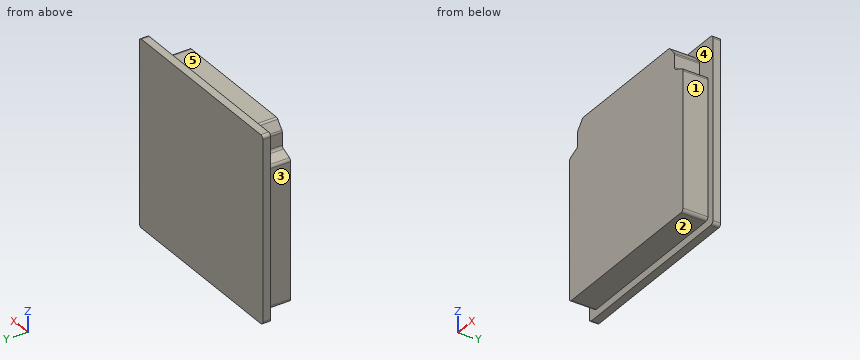
```python
from build123d import *

# Parameters (mm, degrees)
F0_W     = 29.8
F0_H     = 29.8
F1_DEPTH = 1.25
F3_DEPTH = 4
F4_R     = 0.5


with BuildPart() as f1:
    # F0 (on Front) → F1 (new body)
    with BuildSketch(Plane.XZ):
        Rectangle(F0_W, F0_H)
    extrude(amount=F1_DEPTH)

    # F2 (on face) → F3 (join)
    with BuildSketch(Plane.XZ.offset(1.25)):
        Polygon((-13.7, -13.7), (0, -13.7), (13.7, -13.7), (13.7, 8.8), (11.7, 9.7), (11.7, 12.2), (10.45, 13.7), (0, 13.7), (-10.45, 13.7), (-11.7, 12.2), (-11.7, 9.7), (-13.7, 8.8), align=None)
    extrude(amount=F3_DEPTH)

    # F4
    f4_edges = [f1.edges().sort_by_distance(p)[0] for p in [
        (-14.9, -0.625, 14.9),
        (-14.9, -0.625, -14.9),
        (-11.7, -3.25, 12.2),
        (-10.45, -3.25, 13.7),
        (-11.7, -3.25, 9.7),
        (-13.7, -3.25, 8.8),
        (-13.7, -3.25, -13.7),
        (14.9, -0.625, 14.9),
        (14.9, -0.625, -14.9),
        (13.7, -3.25, -13.7),
        (13.7, -3.25, 8.8),
        (11.7, -3.25, 9.7),
        (11.7, -3.25, 12.2),
        (10.45, -3.25, 13.7),
    ]]
    fillet(f4_edges, radius=F4_R)


solid = f1.part
```
Can you work these out from the model? Positions are in its coordinate system, mm. Face numbers are marked on the shaded views. A direction names the side the tool comes from. Give positions to 0.01 mm unless a question says otherwise; leave off trailing zeros. Loops run counter-clockwise (first coordinate to the right, second up) from the corner with the lowest first, then second, coordinate; pieces in that order, holes last. Notation, with made-up numbers: M 34,34.5 L 49,34.5 A22 cw 49,64.5 Z; hole C 6,75 d9. An arc over 180 degrees is marked long. One line per item, written item: value.
(1) I need wall thicknesses on line 1 (Z direction, x = 3.5, y = -3); line 2 (X direction, y = -1.5, z = 10.25). Which ranges of each line are inside material? Lowest first, please.
Returned:
line 1: -13.7 to 13.7
line 2: -11.7 to 11.7
(2) Suppose I cut it at C-C on x = -6.5. List the corners of the cut face in (y, z) for me, plus the area to 3 significant figures.
Returned:
outline: M -5.25,-13.7 L -1.25,-13.7 L -1.25,-14.9 L 0,-14.9 L 0,14.9 L -1.25,14.9 L -1.25,13.7 L -5.25,13.7 Z
area: 147 mm^2
(3) Which directions (+Z, -Z, +X, -X, +Y, -Y) give clear straight access to the entire face, cutting with the end or side of a thin tool? Please do the marked faces 1, 2, 3, 4 and 5.
Returned:
face 1: +Z, -Z, +X, -Y
face 2: -Z, +X, -X, -Y
face 3: +Z, -Z, -X, -Y
face 4: -Y
face 5: +Z, +X, -X, -Y
(4) Will these pins go through, and if not, where does the flat tip stop? pin 1 (1 mm diameter, centred on x = 10, y = -2, fed in from +Z); pin 2 (2 mm diameter, centred on y = -4, z = 2.5, fed in from +X); pin 3 (0.6 mm diameter, centred on y = -3, z = 11, fed in from +X).
Returned:
pin 1: z = 13.7
pin 2: x = 13.7
pin 3: x = 11.7
(5) Suppose I cut it at A-A on z = -7.25. List the corners of the cut face in (x, y) for me.
Returned:
outline: M -14.9,-1.25 L -13.7,-1.25 L -13.7,-5.25 L 13.7,-5.25 L 13.7,-1.25 L 14.9,-1.25 L 14.9,0 L -14.9,0 Z
(6) Suppose I cut it at B-B on y = -2.3. List the corners of the cut face in (x, z) for me.
Returned:
outline: M -13.7,-13.2 A0.5 ccw -13.2,-13.7 L 13.2,-13.7 A0.5 ccw 13.7,-13.2 L 13.7,8.48 A0.5 ccw 13.41,8.93 L 11.99,9.57 A0.5 cw 11.7,10.02 L 11.7,12.02 A0.5 ccw 11.58,12.34 L 10.6,13.52 A0.5 ccw 10.22,13.7 L -10.22,13.7 A0.5 ccw -10.6,13.52 L -11.58,12.34 A0.5 ccw -11.7,12.02 L -11.7,10.02 A0.5 cw -11.99,9.57 L -13.41,8.93 A0.5 ccw -13.7,8.48 Z
